Input: part model. Units: mm. Frame: model coordinates. A direction names the side the tool comes from. Round coordinates to 2 decimals unless told otherwise and drop trailing zeros. Loops run counter-clockwise (first coordinate to the right, second up) from the corner with the lowest first, then second, coordinate; pieces in that order, holes last. Notation, with made-up numbers: (25, 45.25) -> (30, 45.25) arc R33 ccw to (30, 77.25) -> close; hole circle Ø4 at (75.25, -21.5). An arc over 180 degrees is marked (long way). Answer as a JSON object with one key per item and string values.
```python
from build123d import *

# Parameters (mm, degrees)
F0_R     = 12.5
F0_R_2   = 5
F1_DEPTH = 5
F2_DEPTH = 12
F3_DEPTH = 5


with BuildPart() as f1:
    # F0 (on Top) → F1 (new body)
    with BuildSketch(Plane.XY):
        with Locations((5.99056, 3.405503)):
            Circle(F0_R)
        with Locations((5.99056, 3.405503)):
            Circle(F0_R_2, mode=Mode.SUBTRACT)
    extrude(amount=F1_DEPTH)

    # F0 (on Top) → F2 (join)
    with BuildSketch(Plane.XY):
        with BuildLine():
            ThreePointArc((25.99056, 3.405503), (20.132696, 17.547638), (5.99056, 23.405503))
            ThreePointArc((5.99056, 23.405503), (-14.00944, 3.405503), (5.99056, -16.594497))
            ThreePointArc((5.99056, -16.594497), (20.132696, -10.736633), (25.99056, 3.405503))
        make_face()
        with Locations((5.99056, 3.405503)):
            Circle(F0_R, mode=Mode.SUBTRACT)
    extrude(amount=F2_DEPTH)

    # F0 (on Top) → F3 (join)
    with BuildSketch(Plane.XY):
        with BuildLine():
            Line((40.99056, 23.405503), (5.99056, 23.405503))
            ThreePointArc((5.99056, 23.405503), (20.132696, 17.547638), (25.99056, 3.405503))
            ThreePointArc((25.99056, 3.405503), (20.132696, -10.736633), (5.99056, -16.594497))
            Line((5.99056, -16.594497), (40.99056, -16.594497))
            Line((40.99056, -16.594497), (40.99056, 23.405503))
        make_face()
        with BuildLine():
            Line((5.99056, 23.405503), (-29.00944, 23.405503))
            Line((-29.00944, 23.405503), (-29.00944, -16.594497))
            Line((-29.00944, -16.594497), (5.99056, -16.594497))
            ThreePointArc((5.99056, -16.594497), (-14.00944, 3.405503), (5.99056, 23.405503))
        make_face()
    extrude(amount=F3_DEPTH)


solid = f1.part
```
1) Reachability of faces 5 (the face through (17.54, -1.38, 8.45)), 6 (the face through (13, 4, 0)) from +Z, -Z, +X, -X, +Y, -Y: full face, straight path, thin tool, end or side. Return the list, or none.
Output:
{"face 5": "+Z", "face 6": "-Z, +X, -X, +Y, -Y"}
2) Contact query for flat-ended pins moving along their axis: P1, Ø3, axis at x = 20.5, z = 8, coming from the +Y side; P2, Ø1, axis at y = -8.5, z = 8, coming from the +X side; P3, Ø1.5, axis at y = -6, z = 6.5, coming from the -X side; P4, Ø8, axis at x = 5.99, y = 3.41, coming from the +Z side. Output: stop coordinate, or through.
Output:
{"P1": "stops at y = 18.6", "P2": "stops at x = 22.42", "P3": "stops at x = -12.04", "P4": "passes through"}
3) Section B-B, the plane z = 1.25. Output: boundary loops of the cut face in (x, y), plus the area to 3 significant figures.
Output:
{"outline": "(-29.01, -16.59) -> (40.99, -16.59) -> (40.99, 23.41) -> (-29.01, 23.41) -> close; hole circle Ø10 at (5.99, 3.41)", "area": "2,720 mm^2"}
4) Draft query along X for faces 1 (the face through (-29.009, 4, 2)), 2 (the face through (6, -2, 5)), 3 (the face through (8.68, 7.62, 2.46)), 4 (the face through (-20, 4, 5)). Return one class per face: +X half, -X half, draft (parallel to the pull), parting line (faces both ways), or undercut.
Output:
{"face 1": "-X half", "face 2": "undercut", "face 3": "undercut", "face 4": "draft"}
5) Ray query, probe 1 along X at (y, z) = (3.5, 2); probe 2 along Z at (x, y) = (34.5, 2.5); probe 3 along X at (y, z) = (5, 4.5). Return the intervals inside material, ascending.
Output:
{"probe 1": "x = -29.01 to 0.99, 10.99 to 40.99", "probe 2": "z = 0 to 5", "probe 3": "x = -29.01 to 1.25, 10.73 to 40.99"}
6) Section A-A, the plane x = 10. Output: boundary loops of the cut face in (y, z).
Output:
{"outline": "(-16.59, 0) -> (0.42, 0) -> (0.42, 5) -> (-8.43, 5) -> (-8.43, 12) -> (-16.19, 12) -> (-16.19, 5) -> (-16.59, 5) -> close; (6.39, 0) -> (23.41, 0) -> (23.41, 5) -> (23, 5) -> (23, 12) -> (15.25, 12) -> (15.25, 5) -> (6.39, 5) -> close"}
7) Section D-D, the plane x = 35. Output: boundary loops of the cut face in (y, z), plus the area to 3 significant figures.
Output:
{"outline": "(-16.59, 0) -> (23.41, 0) -> (23.41, 5) -> (-16.59, 5) -> close", "area": "200 mm^2"}
8) Section C-C, the plane y = 10. Output: boundary loops of the cut face in (x, z), plus the area to 3 significant figures.
Output:
{"outline": "(-29.01, 0) -> (40.99, 0) -> (40.99, 5) -> (24.87, 5) -> (24.87, 12) -> (16.61, 12) -> (16.61, 5) -> (-4.63, 5) -> (-4.63, 12) -> (-12.89, 12) -> (-12.89, 5) -> (-29.01, 5) -> close", "area": "466 mm^2"}
